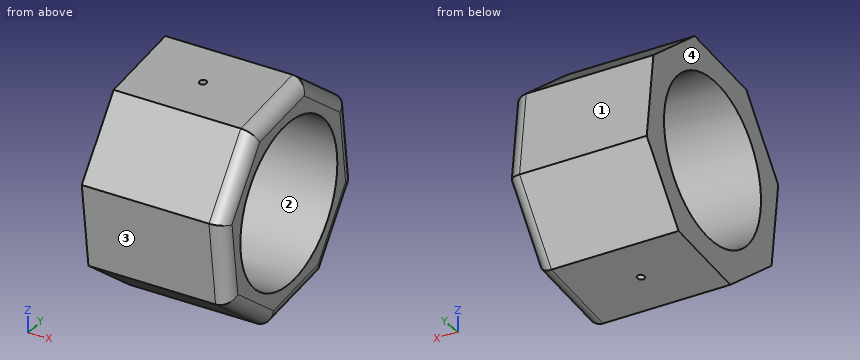
```python
from build123d import *

# Parameters (mm, degrees)
F0_R     = 56.5732299852
F1_DEPTH = 100
F2_R     = 10
F4_D     = 5


with BuildPart() as f1:
    # F0 (on Right) → F1 (new body)
    with BuildSketch(Plane.YZ):
        Polygon((39.5261961416, -68.9136280333), (76.6785350248, -20.7800523723), (68.9136280333, 39.5261961416), (20.7800523723, 76.6785350248), (-39.5261961416, 68.9136280333), (-76.6785350248, 20.7800523723), (-68.9136280333, -39.5261961416), (-20.7800523723, -76.6785350248), align=None)
        Circle(F0_R, mode=Mode.SUBTRACT)
    extrude(amount=F1_DEPTH)

    # F2
    f2_edges = [f1.edges().sort_by_distance(p)[0] for p in [
        (100, -9.373072, 72.796082),
        (100, -58.102366, 44.84684),
        (100, -72.796082, -9.373072),
        (100, -44.84684, -58.102366),
        (100, 9.373072, -72.796082),
        (100, 58.102366, -44.84684),
        (100, 72.796082, 9.373072),
        (100, 44.84684, 58.102366),
    ]]
    fillet(f2_edges, radius=F2_R)

    # F4 (through all)
    with Locations(Plane(origin=(0, 9.3730718847, -72.796081529), x_dir=(1, 0, 0), z_dir=(0, 0.1277036949, -0.9918123645))):
        with Locations((45, 0)):
            Hole(F4_D / 2)


solid = f1.part
```
Can you work these out from the model? Positions are in its coordinate system, mm. Face numbers are marked on the shaded views. Coordinates: 2 decimals unless noted, no trailing zeros. Loops run counter-clockwise (first coordinate to the right, second up) from the corner with the lowest first, then second, coordinate; pieces in that order, holes last. Notation, with made-up numbers: (-35, 59) - (-25, 59) arc R8 cw to (-25, 66) - close; hole circle Ø11 at (15.5, -37). An arc over 180 degrees is marked (long way). Use a Markdown table: item, result.
Item 1: If I drill on probe 1 along Z at (x, y) = (71.5, 0); probe 2 along Y at (x, z) = (8, 36.5); probe 3 along Y at (x, z) = (83, 20), over which ranges is the centre line in solid material (lowest first)? Write a range as from..to.
Numbers:
| item | result |
|---|---|
| probe 1 | z = -74..-56.57, 56.57..74 |
| probe 2 | y = -64.54..-43.22, 43.22..69.3 |
| probe 3 | y = -76.58..-52.92, 52.92..71.43 |
Item 2: We'd pull the mould along Y, two halves only. Please class the marked faces 1, 2, 3 and 4: released by +Y, released by -Y, zero draft, split by the parting line, or undercut.
Numbers:
| item | result |
|---|---|
| face 1 | released by +Y |
| face 2 | undercut |
| face 3 | released by -Y |
| face 4 | zero draft |
Item 3: Will these pins go through, and if not, where does the flat tip stop? pin 1 (10 mm diameter, centred on y = 32, z = -40, fed in from +X); pin 2 (10 mm diameter, centred on x = 74.5, z = 52, fed in from +Y); pin 3 (3 mm diameter, centred on x = 69, y = -26.5, fed in from -Z); pin 4 (6 mm diameter, centred on x = 46.5, z = 37, fed in from +Y).
Numbers:
| item | result |
|---|---|
| pin 1 | passes through |
| pin 2 | stops at y = 59.23 |
| pin 3 | stops at z = -73.42 |
| pin 4 | stops at y = 69.63 |
Item 4: I want a section at A-A on x = 10. Please give me the cut outline in (y, z), and give its area (3 significant figures).
Numbers:
| item | result |
|---|---|
| outline | (-76.68, 20.78) - (-68.91, -39.53) - (-20.78, -76.68) - (39.53, -68.91) - (76.68, -20.78) - (68.91, 39.53) - (20.78, 76.68) - (-39.53, 68.91) - close; hole circle Ø113.15 at (0, 0) |
| area | 7,800 mm2 |
Item 5: I want a section at B-B on x = 92.5. Please give me the cut outline in (y, z), and give its area (3 significant figures).
Numbers:
| item | result |
|---|---|
| outline | (-76.35, 20.69) - (-68.62, -39.36) - (-20.69, -76.35) - (39.36, -68.62) - (76.35, -20.69) - (68.62, 39.36) - (20.69, 76.35) - (-39.36, 68.62) - close; hole circle Ø113.15 at (0, 0) |
| area | 7,640 mm2 |
